from build123d import *

# Parameters (mm, degrees)
BOSS_EXTRUDE1_DEPTH = 74.5
SKETCH2_W           = 1.5
SKETCH2_H           = 149
BOSS_EXTRUDE2_DEPTH = 11


with BuildPart() as part:
    # Sketch1 → Boss-Extrude1 (new, symmetric)
    with BuildSketch(Plane.XY):
        with BuildLine():
            Line((61.819252883, -16.564418887), (60.370364143, -16.176190319))
            ThreePointArc((60.370364143, -16.176190319), (0, -62.5), (-60.370364143, -16.176190319))
            Line((-60.370364143, -16.176190319), (-61.819252883, -16.564418887))
            ThreePointArc((-61.819252883, -16.564418887), (0, -64), (61.819252883, -16.564418887))
        make_face()
    extrude(amount=BOSS_EXTRUDE1_DEPTH, both=True)

    # Sketch2 → Boss-Extrude2 (add)
    with BuildSketch(Plane(origin=(0, 0, 0), x_dir=(0.9659258262890683, 0.25881904510252113, 0), z_dir=(-0.25881904510252113, 0.9659258262890683, 0))):
        with Locations((-63.25, 0)):
            Rectangle(SKETCH2_W, SKETCH2_H)
    extrude(amount=BOSS_EXTRUDE2_DEPTH)


solid = part.part
Geometry: final body of the model. Coordinates: model frame, mm. Give positions to 0.01 mm unless a question says otherwise; leave off trailing zeros. Write each loop counter-clockwise with the first axis right and the second up, starting at its lowest first coordinate (ties: lowest second). Pieces come first, ordered by that corner, then holes. Notation, with made-up numbers: (19.25, 52) - (73.25, 52) arc R31 cw to (73.25, 83) - close; hole circle Ø10 at (45.25, 82). An arc over 180 degrees is marked (long way). Return JSON: item names as keys, results as strings. Group by question number.
1) Section B-B on z = -8. Return the cut outline in (x, y).
2) First-contact query: P1, Ø2, axis at y = -16, z = -23.5, coming from the -X side; P2, Ø10, axis at y = -13.5, z = 6, coming from the -X side; P3, Ø4, axis at y = -56, z = -24.5, coming from the +X side; P4, Ø1.5, axis at x = 48.5, y = -42.5, coming from the -Z side. Flat tips, straight axial feed; report the tip coordinate or a pass-through.
3) Section A-A on y = -23. Return the cut outline in (x, z).
4) Mould query, pull axis X, two halves, no side actions, for faces 1 (the flat face through (8, -63, -74.5)), 2 (the cylindrical face through (-1.17, -63.99, 1.04)), 3 (the cylindrical face through (1.15, -62.49, 1.04)). Classes: released by +X, released by -X, zero draft, split by the parting line, or undercut.
5) Line query: line 1 (X direction, y = -33, z = -31); line 2 (X direction, y = -32, z = 12); line 3 (Y direction, x = -57, z = -50). Output: solid intervals per line, ascending.
6) Section D-D on x = 15.5. Return the cut outline in (y, z), plus the area to 3 significant figures.
Filled in:
{
 "1": {"outline": "(-64.67, -5.94) - (-61.82, -16.56) arc R64 ccw to (61.82, -16.56) - (60.37, -16.18) arc R62.5 cw to (-60.37, -16.18) - (-63.22, -5.55) - close"},
 "2": {"P1": "stops at x = -62.24", "P2": "stops at x = -63.98", "P3": "stops at x = 34.35", "P4": "stops at z = -74.5"},
 "3": {"outline": "(-59.72, -74.5) - (-58.11, -74.5) - (-58.11, 74.5) - (-59.72, 74.5) - close; (58.11, -74.5) - (59.72, -74.5) - (59.72, 74.5) - (58.11, 74.5) - close"},
 "4": {"face 1": "zero draft", "face 2": "split by the parting line", "face 3": "undercut"},
 "5": {"line 1": "x = -54.84 to -53.08, 53.08 to 54.84", "line 2": "x = -55.43 to -53.69, 53.69 to 55.43", "line 3": "y = -29.1 to -25.64"},
 "6": {"outline": "(-62.09, -74.5) - (-60.55, -74.5) - (-60.55, 74.5) - (-62.09, 74.5) - close", "area": "231 mm^2"}
}
